Could you check a few things on this model? Use its own coordinates, in mm. A direction names the side the tool comes from. Give positions to 0.01 mm unless a question says otherwise; leave off trailing zeros. Order: outer loops, then holes, each group sorted by start corner. A loop starts at its lowest first (then second) coordinate and runs counter-clockwise, first axis right, second up. Notation, with made-up numbers: (-35, 7.5) - (8, 7.5) arc R19 ccw to (8, 39.5) - close; hole circle Ø10 at (82.25, 12.5). An arc over 180 degrees is marked (long way). One line per question, with ' | ' between items. Start each with the question number.
1. I need wall thicknesses on probe 1 along Z at (x, y) = (0, 21.5); probe 2 along X at (y, z) = (0.5, 700) (3 decimals); probe 3 along Y at (x, z) = (-0.5, 92.5) (3 decimals). Which ranges of each line are inside material? Lowest first, please. Write a range as from..to.
2. If we mould it in two halves opening along Z, with no side actions, what happens to faces 6 (the flat face through (-22, 66, 698)), 7 (the flat face through (-8, -25, 730)), 8 (the flat face through (-22.34, 3.82, 783))? For each: released by +Z, released by -Z, zero draft, split by the parting line, or undercut.
3. Imagine slicing it at B-B (y = 46). Please give me the cut outline in (x, z), and give its area (3 significant figures).
4. Which directions (+Z, -Z, +X, -X, +Y, -Y) give clear straight access to the entire face, cutting with the end or side of a thin tool? Please do faces 1 (the cylindrical face through (-20.784, 44.957, 691.382)), 2 (the flat face through (0, 0, 730)), 3 (the cylindrical face through (0.1, -24.4, 85)), 4 (the cylindrical face through (23.846, 7.509, 757.65)), 5 (the flat face through (-9.4, 22.3, 0)).
5. For P1, Ø8, axis at y = 6, z = 492.5, coming from the +X side; P2, Ø12, axis at x = -3.5, z = 669.5, coming from the -Y side; P3, Ø1, axis at y = -6.5, z = 201, coming from the +X side, each with a flat end and sliding along its axis, tell me the tip position at first contact or that it passes through.
6. Imagine slicing it at D-D (x = -11). Give the number of separate pieces and of enclosed holes in the cut face, and give its area (3 significant figures).
7. Imagine slicing it at A-A (y = 0). Please give me the cut outline in (x, z).
8. Imagine slicing it at C-C (z = 749). Please give me the cut outline in (x, y).
```python
from build123d import *

# Parameters (mm, degrees)
F1_R      = 25
F1_R_2    = 24
F4_DEPTH  = 27.5
F5_R      = 25
F6_DEPTH  = 50
F7_R      = 22.5
F8_DEPTH  = 55
F9_R      = 21.5
F10_DEPTH = 20
F9_R_2    = 22.5
F11_DEPTH = 38.5
F13_DEPTH = 38.5


with BuildPart() as f2:
    # F2: sweep along a path in F0
    with BuildLine(Plane.YZ) as f2_path:
        Line((0, 0), (0, 730))
    # F1 (on Top) → F2 (sweep)
    with BuildSketch(Plane.XY):
        Circle(F1_R)
        Circle(F1_R_2, mode=Mode.SUBTRACT)
    sweep(path=f2_path.line)

    # F3 (on Right) → F4 (join, symmetric)
    with BuildSketch(Plane.YZ):
        Polygon((-27.5, 730), (-25, 730), (25, 730), (27.5, 730), (27.5, 733), (-27.5, 733), align=None)
    extrude(amount=F4_DEPTH, both=True)

    # F5 (on face) → F6 (join)
    with BuildSketch(Plane.XY.offset(733)):
        Circle(F5_R)
    extrude(amount=F6_DEPTH)

    # F7 (on face) → F8 (join)
    with BuildSketch(Plane.XY.offset(783)):
        Circle(F7_R)
    extrude(amount=F8_DEPTH)

    # F9 (on face) → F10 (cut)
    with BuildSketch(Plane(origin=(0, 27.5, 0), x_dir=(-1, 0, 0), z_dir=(0, 1, 0))):
        with Locations((0, 700)):
            Circle(F9_R)
    extrude(amount=-F10_DEPTH, mode=Mode.SUBTRACT)

    # F9 (on face) → F11 (join, symmetric)
    with BuildSketch(Plane(origin=(0, 27.5, 0), x_dir=(-1, 0, 0), z_dir=(0, 1, 0))):
        with Locations((0, 700)):
            Circle(F9_R_2)
        with Locations((0, 700)):
            Circle(F9_R, mode=Mode.SUBTRACT)
    extrude(amount=F11_DEPTH, both=True)

    # F12 (on face) → F13 (cut)
    with BuildSketch(Plane.XZ.offset(27.5)):
        with BuildLine():
            Line((-20, 65), (-20, 25))
            ThreePointArc((-20, 25), (0, 5), (20, 25))
            Line((20, 25), (20, 65))
            ThreePointArc((20, 65), (0, 85), (-20, 65))
        make_face()
    extrude(amount=-F13_DEPTH, mode=Mode.SUBTRACT)


solid = f2.part
```
Results found:
1) probe 1: z = 677.5..678.5, 721.5..722.5, 730..838 | probe 2: x = -24.995..-23.995, -22.5..-21.5, 21.5..22.5, 23.995..24.995 | probe 3: y = -24.995..-23.995, 23.995..24.995
2) face 6: zero draft | face 7: undercut | face 8: released by +Z
3) outline: circle Ø45 at (0, 700); hole circle Ø43 at (0, 700) | area: 138 mm2
4) face 1: +Y | face 2: none | face 3: -Y | face 4: +Z | face 5: -Z, +X, -X, +Y, -Y
5) P1: stops at x = 24.92 | P2: stops at y = -25 | P3: stops at x = 24.27
6) separate pieces: 3 | enclosed holes: 0 | area: 6,250 mm2
7) outline: (-27.5, 730) - (-25, 730) - (-25, 0) - (-24, 0) - (-24, 730) - (24, 730) - (24, 0) - (25, 0) - (25, 730) - (27.5, 730) - (27.5, 733) - (25, 733) - (25, 783) - (22.5, 783) - (22.5, 838) - (-22.5, 838) - (-22.5, 783) - (-25, 783) - (-25, 733) - (-27.5, 733) - close; circle Ø45 at (0, 700); hole circle Ø43 at (0, 700)
8) outline: circle Ø50 at (0, 0)
